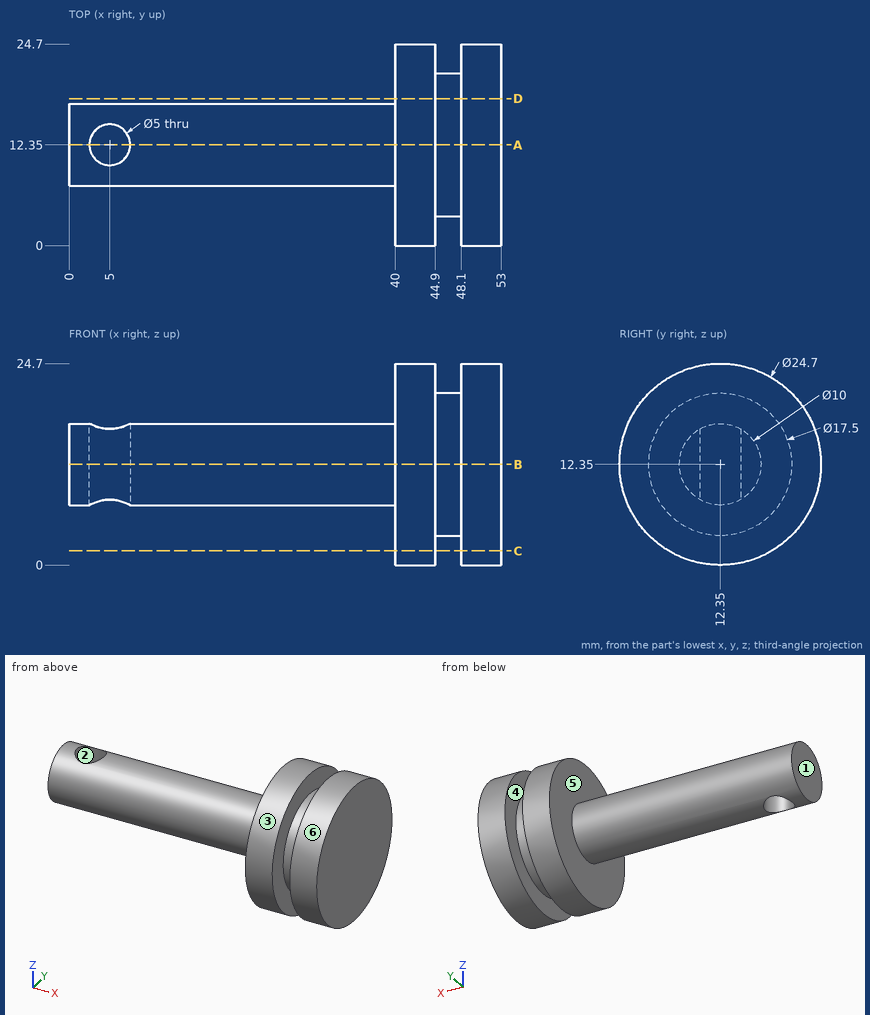
Drawing for the job (mm, zero at the part's lowest x, y, z). A direction names the side the tool comes from. Give positions to 0.01 mm unless a question says otherwise; leave off trailing zeros. Write each loop counter-clockwise with the first axis right and the second up, starting at its lowest first coordinate (ties: lowest second). Pieces come first, ordered by that corner, then holes. Notation, with made-up numbers: M -11,29 L 19,29 A9 cw 19,44 Z; hole C -32,76.25 d11. An arc over 180 degrees is marked long. Use CSV: the item, a comma, the result in double quotes.
Item 1: Pull direction Y, two halves, no side cores. Call the marked faces 1, 2 and 3: +Y half, -Y half, draft (parallel to the pull), parting line (faces both ways), or undercut.
Taken from the geometry:
face 1,"draft"
face 2,"undercut"
face 3,"parting line"
Item 2: Which spindle directions (+Z, -Z, +X, -X, +Y, -Y) get a long thin tool onto all of the face, cutting with end or side? Do the marked faces 4, 5 and 6. Say none if no direction does.
Taken from the geometry:
face 4,"none"
face 5,"-X"
face 6,"+X, -X"
Item 3: Slice it at A-A on y = 12.35. Write the cut outline in (x, z), plus the area to 3 significant figures.
Taken from the geometry:
outline,"M 0,7.35 L 2.5,7.35 L 2.5,17.35 L 0,17.35 Z; M 7.5,7.35 L 40,7.35 L 40,0 L 44.9,0 L 44.9,3.6 L 48.1,3.6 L 48.1,0 L 53,0 L 53,24.7 L 48.1,24.7 L 48.1,21.1 L 44.9,21.1 L 44.9,24.7 L 40,24.7 L 40,17.35 L 7.5,17.35 Z"
area,"648 mm²"
Item 4: Slice it at B-B on z = 12.35. Write the cut outline in (x, y).
Taken from the geometry:
outline,"M 0,7.35 L 40,7.35 L 40,0 L 44.9,0 L 44.9,3.6 L 48.1,3.6 L 48.1,0 L 53,0 L 53,24.7 L 48.1,24.7 L 48.1,21.1 L 44.9,21.1 L 44.9,24.7 L 40,24.7 L 40,17.35 L 0,17.35 Z; hole C 5,12.35 d5"
Item 5: Slice it at C-C on z = 1.75. Write the cut outline in (x, y), plus the area to 3 significant figures.
Taken from the geometry:
outline,"M 40,6.01 L 44.9,6.01 L 44.9,18.69 L 40,18.69 Z; M 48.1,6.01 L 53,6.01 L 53,18.69 L 48.1,18.69 Z"
area,"124 mm²"
Item 6: Slice it at D-D on y = 18. Write the cut outline in (x, z), plus the area to 3 significant figures.
Taken from the geometry:
outline,"M 40,1.37 L 44.9,1.37 L 44.9,5.67 L 48.1,5.67 L 48.1,1.37 L 53,1.37 L 53,23.33 L 48.1,23.33 L 48.1,19.03 L 44.9,19.03 L 44.9,23.33 L 40,23.33 Z"
area,"258 mm²"
Item 7: Drill centre lines: probe 1 along X at (y, z) = (23.25, 11.5); probe 2 along X at (y, z) = (12.35, 11.5); probe 3 along Y at (x, z) = (5, 11). Where is each one in solid material? Low to high.
Taken from the geometry:
probe 1,"x = 40 to 44.9, 48.1 to 53"
probe 2,"x = 0 to 2.5, 7.5 to 53"
probe 3,"y = 7.54 to 9.85, 14.85 to 17.16"
Item 8: Pin check, flat tips, straight feed: P1, Ø5, axis at y = 22, z = 19, coming from the -X side; P2, Ø8, axis at x = 15, y = 19.5, coming from the +Z side; P3, Ø8, axis at x = 40, z = 9, coming from the -Y side; P4, Ø12, axis at x = 11, y = 12, coming from the +Z side. Stop position of each tip, or through.
Taken from the geometry:
P1,"stops at x = 40"
P2,"stops at z = 16.23"
P3,"stops at y = 0"
P4,"stops at z = 17.35"
